from build123d import *

# Parameters (mm, degrees)
SKETCH1_W                          = 139.7
SKETCH1_H                          = 25.4
BOSS_EXTRUDE1_DEPTH                = 3.175
CUT_EXTRUDE1_REACH                 = 73.279
SKETCH2_W                          = 6.35
SKETCH2_H                          = 5.08
TAP_DRILL_FOR_8_32_TAP1_AT_2_COUNT = 2
TAP_DRILL_FOR_8_32_TAP1_AT_2_PITCH = 47.625
TAP_DRILL_FOR_8_32_TAP1_AT_3_COUNT = 2
TAP_DRILL_FOR_8_32_TAP1_AT_3_PITCH = 85.725
TAP_DRILL_FOR_8_32_TAP1_AT_4_COUNT = 2
TAP_DRILL_FOR_8_32_TAP1_AT_4_PITCH = 133.35


with BuildPart() as part:
    # Sketch1 → Boss-Extrude1 (new, symmetric)
    with BuildSketch(Plane.XY):
        Rectangle(SKETCH1_W, SKETCH1_H)
    extrude(amount=BOSS_EXTRUDE1_DEPTH, both=True)

    # Sketch2 → Cut-Extrude1 (cut, up to next)
    with BuildSketch(Plane.XY.offset(3.175), mode=Mode.PRIVATE) as cut_extrude1_sk1:
        with Locations((-66.675, 10.16)):
            Rectangle(SKETCH2_W, SKETCH2_H)
    cut_extrude1_tool1 = extrude(cut_extrude1_sk1.sketch, amount=-CUT_EXTRUDE1_REACH, mode=Mode.PRIVATE) & part.part
    # Sketch2 → Cut-Extrude1 (cut, up to next)
    with BuildSketch(Plane.XY.offset(3.175), mode=Mode.PRIVATE) as cut_extrude1_sk2:
        with Locations((-66.675, -10.16)):
            Rectangle(SKETCH2_W, SKETCH2_H)
    cut_extrude1_tool2 = extrude(cut_extrude1_sk2.sketch, amount=-CUT_EXTRUDE1_REACH, mode=Mode.PRIVATE) & part.part
    # Sketch2 → Cut-Extrude1 (cut, up to next)
    with BuildSketch(Plane.XY.offset(3.175), mode=Mode.PRIVATE) as cut_extrude1_sk3:
        with Locations((66.675, 10.16)):
            Rectangle(SKETCH2_W, SKETCH2_H)
    cut_extrude1_tool3 = extrude(cut_extrude1_sk3.sketch, amount=-CUT_EXTRUDE1_REACH, mode=Mode.PRIVATE) & part.part
    # Sketch2 → Cut-Extrude1 (cut, up to next)
    with BuildSketch(Plane.XY.offset(3.175), mode=Mode.PRIVATE) as cut_extrude1_sk4:
        with Locations((66.675, -10.16)):
            Rectangle(SKETCH2_W, SKETCH2_H)
    cut_extrude1_tool4 = extrude(cut_extrude1_sk4.sketch, amount=-CUT_EXTRUDE1_REACH, mode=Mode.PRIVATE) & part.part
    add(cut_extrude1_tool1.solids().sort_by_distance((-66.675, 10.16, 3.175))[0], mode=Mode.SUBTRACT)
    add(cut_extrude1_tool2.solids().sort_by_distance((-66.675, -10.16, 3.175))[0], mode=Mode.SUBTRACT)
    add(cut_extrude1_tool3.solids().sort_by_distance((66.675, 10.16, 3.175))[0], mode=Mode.SUBTRACT)
    add(cut_extrude1_tool4.solids().sort_by_distance((66.675, -10.16, 3.175))[0], mode=Mode.SUBTRACT)

    # Sketch5 → Tap Drill for #8-32 Tap1 (revolve, cut)
    with BuildSketch(Plane(origin=(-66.675, 12.7, 0), x_dir=(0, 0, 1), z_dir=(1, 0, 0))):
        Polygon((0, 0), (0, 13.737806461), (1.7272, 12.7), (1.7272, 0), align=None)
    tap_drill_for_8_32_tap1 = revolve(axis=Axis((-66.675, 19.05, 0), (0, -1, 0)), mode=Mode.SUBTRACT)

    # Tap Drill for #8-32 Tap1 at 2: Tap Drill for #8-32 Tap1 ×2
    with Locations(*[(i * TAP_DRILL_FOR_8_32_TAP1_AT_2_PITCH, 0, 0) for i in range(1, TAP_DRILL_FOR_8_32_TAP1_AT_2_COUNT)]):
        add(tap_drill_for_8_32_tap1, mode=Mode.SUBTRACT)

    # Tap Drill for #8-32 Tap1 at 3: Tap Drill for #8-32 Tap1 ×2
    with Locations(*[(i * TAP_DRILL_FOR_8_32_TAP1_AT_3_PITCH, 0, 0) for i in range(1, TAP_DRILL_FOR_8_32_TAP1_AT_3_COUNT)]):
        add(tap_drill_for_8_32_tap1, mode=Mode.SUBTRACT)

    # Tap Drill for #8-32 Tap1 at 4: Tap Drill for #8-32 Tap1 ×2
    with Locations(*[(i * TAP_DRILL_FOR_8_32_TAP1_AT_4_PITCH, 0, 0) for i in range(1, TAP_DRILL_FOR_8_32_TAP1_AT_4_COUNT)]):
        add(tap_drill_for_8_32_tap1, mode=Mode.SUBTRACT)

    # Mirror1: Tap Drill for #8-32 Tap1 across plane
    add(tap_drill_for_8_32_tap1.mirror(Plane.ZX), mode=Mode.SUBTRACT)

    # Mirror1 copy 1 sketch → Mirror1 copy 1 (revolve, cut)
    with BuildSketch(Plane(origin=(-19.05, -12.7, 0), x_dir=(0, 0, 1), z_dir=(1, 0, 0))):
        Polygon((0, 0), (0, -13.737806461), (1.7272, -12.7), (1.7272, 0), align=None)
    revolve(axis=Axis((-19.05, -19.05, 0), (0, -1, 0)), mode=Mode.SUBTRACT)

    # Mirror1 copy 2 sketch → Mirror1 copy 2 (revolve, cut)
    with BuildSketch(Plane(origin=(19.05, -12.7, 0), x_dir=(0, 0, 1), z_dir=(1, 0, 0))):
        Polygon((0, 0), (0, -13.737806461), (1.7272, -12.7), (1.7272, 0), align=None)
    revolve(axis=Axis((19.05, -19.05, 0), (0, -1, 0)), mode=Mode.SUBTRACT)

    # Mirror1 copy 3 sketch → Mirror1 copy 3 (revolve, cut)
    with BuildSketch(Plane(origin=(66.675, -12.7, 0), x_dir=(0, 0, 1), z_dir=(1, 0, 0))):
        Polygon((0, 0), (0, -13.737806461), (1.7272, -12.7), (1.7272, 0), align=None)
    revolve(axis=Axis((66.675, -19.05, 0), (0, -1, 0)), mode=Mode.SUBTRACT)


solid = part.part
Verification items for the finished model (mm, model axes). A direction names the side the tool comes from. Round coordinates to 2 decimals unless told otherwise and drop trailing zeros. Write each loop counter-clockwise with the first axis right and the second up, starting at its lowest first coordinate (ties: lowest second). Pieces come first, ordered by that corner, then holes.
(1) Access from +Z, -Z, +X, -X, +Y, -Y to the whole of each face (thin tool, end or side, straight path). Record for faces 5 (the flat face through (63.5, 10, 0)), 6 (the flat face through (-68.1, -7.62, -1.4)), 7 (the flat face through (65, -7.62, -1)), 8 (the flat face through (-68.1, 7.62, -1.4)).
Returned:
face 5: +Z, -Z, +X, +Y
face 6: +Z, -Z, -X, -Y
face 7: +Z, -Z, +X, -Y
face 8: +Z, -Z, -X, +Y
(2) Section check C-C (y = -1.5). Enter the section's corners in (x, z) (3 decimals).
Returned:
outline: (-69.85, -3.175) - (69.85, -3.175) - (69.85, 3.175) - (-69.85, 3.175) - close; hole circle Ø3.454 at (-66.675, 0); hole circle Ø3.454 at (-19.05, 0); hole circle Ø3.454 at (19.05, 0); hole circle Ø3.454 at (66.675, 0)
(3) Mould release check, pull along Z, two halves, no side actions. Record for faces 1 (the cylindrical face through (-68.39, -0.11, -0.22)), 2 (the flat face through (-1, 0, -3.175)), 3 (the flat face through (-63.5, -10, 0)), 4 (the flat face through (-1, 0, 3.175)): pulls with the +Z half, pulls with the -Z half, needs draft (parallel to the pull), parting line crosses it, or undercut.
Returned:
face 1: undercut
face 2: pulls with the -Z half
face 3: needs draft
face 4: pulls with the +Z half
(4) Depth check by flat-ended pin: pin 1 Ø3 at (x, z) = (-68.5, -1.5) entering from +Y; pin 2 Ø2.5 at (y, z) = (9, 0.5) entering from +X; pin 3 Ø3 at (x, z) = (-67.5, -1) entering from -Y. Enter the tip coordinate at first touch or a pass-through.
Returned:
pin 1: stops at y = 7.62
pin 2: stops at x = 63.5
pin 3: stops at y = -7.62
(5) Section check A-A (z = 0). Enter the section's corners in (x, y).
Returned:
outline: (-69.85, -7.62) - (-68.4, -7.62) - (-68.4, 7.62) - (-69.85, 7.62) - close; (-64.95, -7.62) - (-63.5, -7.62) - (-63.5, -12.7) - (-20.78, -12.7) - (-20.78, 12.7) - (-63.5, 12.7) - (-63.5, 7.62) - (-64.95, 7.62) - close; (-17.32, -12.7) - (17.32, -12.7) - (17.32, 12.7) - (-17.32, 12.7) - close; (20.78, -12.7) - (63.5, -12.7) - (63.5, -7.62) - (64.95, -7.62) - (64.95, 7.62) - (63.5, 7.62) - (63.5, 12.7) - (20.78, 12.7) - close; (68.4, -7.62) - (69.85, -7.62) - (69.85, 7.62) - (68.4, 7.62) - close
(6) Section check B-B (x = -19.05). Enter the section's corners in (y, z) (3 decimals), plus the area to 3 significant figures.
Returned:
outline: (-12.7, -3.175) - (12.7, -3.175) - (12.7, -1.727) - (-12.7, -1.727) - close; (-12.7, 1.727) - (12.7, 1.727) - (12.7, 3.175) - (-12.7, 3.175) - close
area: 73.5 mm2
(7) Material ranges on line 1 (X direction, y = -7.25, z = 0); line 2 (Z direction, x = -19.05, y = -8) (3 decimals); line 3 (X direction, y = 6.25, z = 1), recorded low to high.
Returned:
line 1: x = -69.85 to -68.4, -64.95 to -20.78, -17.32 to 17.32, 20.78 to 64.95, 68.4 to 69.85
line 2: z = -3.175 to -1.727, 1.727 to 3.175
line 3: x = -69.85 to -68.08, -65.27 to -20.46, -17.64 to 17.64, 20.46 to 65.27, 68.08 to 69.85
